Read the model definition and answer for the solid it produces. Units are mm, in the model's axes. A direction names the side the tool comes from. Coordinates: 2 decimals unless noted, no trailing zeros. Write each loop counter-clockwise with the first axis right and the second up, starting at its lowest first coordinate (ties: lowest second). Pieces come first, ordered by that corner, then holes. Notation, with made-up numbers: M 70,26 L 78,26 A13 cw 78,41 Z; hole C 13,76.5 d7. An arc over 180 degrees is marked long. Write item = value, one per line.
from build123d import *

# Parameters (mm, degrees)
BOSS_EXTRUDE1_DEPTH = 5
CUT_EXTRUDE1_DEPTH  = 42.207887594
CUT_EXTRUDE2_REACH  = 43.822
SKETCH5_R           = 1.5
SKETCH6_W           = 0.6
SKETCH6_H           = 2
CUT_EXTRUDE3_DEPTH  = 0.6
SKETCH8_W           = 56.6
SKETCH8_H           = 2.4
BOSS_EXTRUDE2_DEPTH = 2
SKETCH9_W           = 45
SKETCH9_H           = 5
BOSS_EXTRUDE3_DEPTH = 3
FILLET1_START       = -3
FILLET1_DEPTH       = 10
FILLET1_2_DEPTH     = 3
FILLET2_R           = 1


with BuildPart() as part:
    # Sketch1 → Boss-Extrude1 (new, symmetric)
    with BuildSketch(Plane.XY):
        with BuildLine():
            Line((-26.3, 1), (-26.3, 0))
            Line((-26.3, 0), (26.3, 0))
            Line((26.3, 0), (26.3, 1))
            ThreePointArc((26.3, 1), (28.057359313, 5.242640687), (32.3, 7))
            Line((32.3, 7), (40.3, 7))
            Line((40.3, 7), (40.3, 4))
            Line((40.3, 4), (32.3, 4))
            ThreePointArc((32.3, 4), (30.178679656, 3.121320344), (29.3, 1))
            Line((29.3, 1), (29.3, -2))
            ThreePointArc((29.3, -2), (29.007106781, -2.707106781), (28.3, -3))
            Line((28.3, -3), (-28.3, -3))
            ThreePointArc((-28.3, -3), (-29.007106781, -2.707106781), (-29.3, -2))
            Line((-29.3, -2), (-29.3, 1))
            ThreePointArc((-29.3, 1), (-30.178679656, 3.121320344), (-32.3, 4))
            Line((-32.3, 4), (-40.3, 4))
            Line((-40.3, 4), (-40.3, 7))
            Line((-40.3, 7), (-32.3, 7))
            ThreePointArc((-32.3, 7), (-28.057359313, 5.242640687), (-26.3, 1))
        make_face()
    extrude(amount=BOSS_EXTRUDE1_DEPTH, both=True)

    # Sketch3 → Cut-Extrude1 (cut, through all)
    with BuildSketch(Plane(origin=(0, 0, 0), x_dir=(1, 0, 0), z_dir=(0, 1, 0))):
        with BuildLine():
            Line((-23.6, 1.4), (23.6, 1.4))
            ThreePointArc((23.6, 1.4), (25, 0), (23.6, -1.4))
            Line((23.6, -1.4), (-23.6, -1.4))
            ThreePointArc((-23.6, -1.4), (-25, 0), (-23.6, 1.4))
        make_face()
    extrude(amount=-CUT_EXTRUDE1_DEPTH, mode=Mode.SUBTRACT)

    # Sketch5 → Cut-Extrude2 (cut, up to next)
    with BuildSketch(Plane(origin=(0, 7, 0), x_dir=(1, 0, 0), z_dir=(0, 1, 0)), mode=Mode.PRIVATE) as cut_extrude2_sk1:
        with Locations(Location((-36.3, 0, 0), (0, 0, 180))):
            Circle(SKETCH5_R)
    cut_extrude2_tool1 = extrude(cut_extrude2_sk1.sketch, amount=-CUT_EXTRUDE2_REACH, mode=Mode.PRIVATE) & part.part
    # Sketch5 → Cut-Extrude2 (cut, up to next)
    with BuildSketch(Plane(origin=(0, 7, 0), x_dir=(1, 0, 0), z_dir=(0, 1, 0)), mode=Mode.PRIVATE) as cut_extrude2_sk2:
        with Locations(Location((36.3, 0, 0), (0, 0, 180))):
            Circle(SKETCH5_R)
    cut_extrude2_tool2 = extrude(cut_extrude2_sk2.sketch, amount=-CUT_EXTRUDE2_REACH, mode=Mode.PRIVATE) & part.part
    add(cut_extrude2_tool1.solids().sort_by_distance((-36.3, 7, 0))[0], mode=Mode.SUBTRACT)
    add(cut_extrude2_tool2.solids().sort_by_distance((36.3, 7, 0))[0], mode=Mode.SUBTRACT)

    # Sketch6 → Cut-Extrude3 (cut)
    with BuildSketch(Plane(origin=(0, 0, 0), x_dir=(1, 0, 0), z_dir=(0, 1, 0))):
        with Locations((-5.9, 4)):
            Rectangle(SKETCH6_W, SKETCH6_H)
        with Locations((-3.4, 4)):
            Rectangle(SKETCH6_W, SKETCH6_H)
        with Locations((3.4, 4)):
            Rectangle(SKETCH6_W, SKETCH6_H)
        with Locations((-8.4, 4)):
            Rectangle(SKETCH6_W, SKETCH6_H)
        with Locations((-10.9, 4)):
            Rectangle(SKETCH6_W, SKETCH6_H)
        with Locations((-13.4, 4)):
            Rectangle(SKETCH6_W, SKETCH6_H)
        with Locations((5.9, 4)):
            Rectangle(SKETCH6_W, SKETCH6_H)
        with Locations((8.4, 4)):
            Rectangle(SKETCH6_W, SKETCH6_H)
        with Locations((10.9, 4)):
            Rectangle(SKETCH6_W, SKETCH6_H)
        with Locations((13.4, 4)):
            Rectangle(SKETCH6_W, SKETCH6_H)
    extrude(amount=-CUT_EXTRUDE3_DEPTH, mode=Mode.SUBTRACT)

    # Sketch8 → Boss-Extrude2 (add)
    with BuildSketch(Plane.XZ.offset(3)):
        with Locations((0, 3.8)):
            Rectangle(SKETCH8_W, SKETCH8_H)
    extrude(amount=BOSS_EXTRUDE2_DEPTH)

    # Sketch9 → Boss-Extrude3 (add)
    with BuildSketch(Plane.XZ.offset(3)):
        with Locations((0, -7.5)):
            Rectangle(SKETCH9_W, SKETCH9_H)
    extrude(amount=-BOSS_EXTRUDE3_DEPTH)

    # Fillet1: read off the stored shape, not the designer's step
    # Fillet1 outline → Fillet1 (cut)
    with BuildSketch(Plane(origin=(0, 0, 0), x_dir=(1, 0, 0), z_dir=(0, 1, 0)).offset(FILLET1_START)):
        with BuildLine():
            Line((-22.5, 10), (-22.5, 7.5))
            ThreePointArc((-22.5, 7.5), (-21.767766953, 9.267766953), (-20, 10))
            Line((-20, 10), (-22.5, 10))
        make_face()
        with BuildLine():
            Line((22.5, 10), (20, 10))
            ThreePointArc((20, 10), (21.767766953, 9.267766953), (22.5, 7.5))
            Line((22.5, 7.5), (22.5, 10))
        make_face()
    extrude(amount=FILLET1_DEPTH, mode=Mode.SUBTRACT)

    # Fillet1 2 outline → Fillet1 2 (add)
    with BuildSketch(Plane(origin=(0, 0, 0), x_dir=(1, 0, 0), z_dir=(0, 1, 0)).offset(FILLET1_START)):
        with BuildLine():
            Line((-22.5, 5), (-22.5, 7.5))
            ThreePointArc((-22.5, 7.5), (-23.232233047, 5.732233047), (-25, 5))
            Line((-25, 5), (-22.5, 5))
        make_face()
        with BuildLine():
            ThreePointArc((25, 5), (23.232233047, 5.732233047), (22.5, 7.5))
            Line((22.5, 7.5), (22.5, 5))
            Line((22.5, 5), (25, 5))
        make_face()
    extrude(amount=FILLET1_2_DEPTH)

    # Fillet2
    fillet2_edges = [part.edges().sort_by_distance(p)[0] for p in [
        (-28.3, -5, 3.8),
        (28.3, -5, 3.8),
    ]]
    fillet(fillet2_edges, radius=FILLET2_R)


solid = part.part
Item 1: Find section C-C (y = 1.75). Determine the outline of the cut face in (x, z).
Worked answers:
outline = M -29.4,-5 L -26.35,-5 L -26.35,5 L -29.4,5 Z; M 26.35,-5 L 29.4,-5 L 29.4,5 L 26.35,5 Z
Item 2: Which of the six approach directions +Z, -Z, +X, -X, +Y, -Y give full straight-line access (tool end or side, diameter ignored) to faces 4 (the face through (-34, 4, 0)), 5 (the face through (32.8, 4.3, -5)), 6 (the face through (-31, 4, -5))?
Worked answers:
face_4 = +Z, -Z, -X, -Y
face_5 = -Z, +X, +Y, -Y
face_6 = -Z, -X, +Y, -Y
Item 3: Find section B-B (z = 0). State how many separate pieces and enclosed holes the cut face has, and give its area (3 significant figures).
Worked answers:
separate_pieces = 4
enclosed_holes = 0
area = 104 mm²
Item 4: Find section A-A (x = 36.3). Determine the outline of the cut face in (y, z).
Worked answers:
outline = M 4,-5 L 7,-5 L 7,-1.5 L 4,-1.5 Z; M 4,1.5 L 7,1.5 L 7,5 L 4,5 Z
Item 5: Flat-ended cylindrical pins translate along their axes: pin 1 (6 mm diameter, centred on x = -14, z = 1.5, fed in from -Y); pin 2 (1.1 mm diameter, centred on y = 0.5, z = -2, fed in from -X); pin 3 (2.5 mm diameter, centred on x = 35.5, z = -1.5, fed in from -Y); pin 4 (6 mm diameter, centred on y = -1, z = -1, fed in from -X). Find the tip coordinate at first contact, or state that the pin passes through.
Worked answers:
pin_1 = -5
pin_2 = -29.3
pin_3 = 4
pin_4 = -29.47
Item 6: Consider line 1 along Z through (x, y) = (36.3, 4.85); line 2 along Y through (x, z) = (37, 2.25); line 3 along X through (y, z) = (0.75, 2). Determine where each line is inside the solid, lowest interval first. Write a range as from..to.
Worked answers:
line_1 = -5..-1.5, 1.5..5
line_2 = 4..7
line_3 = -29.3..-26.3, 26.3..29.3
Item 7: Find section D-D (x = -4.5). Determine the outline of the cut face in (y, z), and give its area (3 significant figures).
Worked answers:
outline = M -5,2.6 L -3,2.6 L -3,1.4 L 0,1.4 L 0,5 L -5,5 Z; M -3,-10 L 0,-10 L 0,-1.4 L -3,-1.4 Z
area = 41.4 mm²
Item 8: For a pull along Z with two mould halves and no side action, classify faces 1 (the face through (-40.3, 5, 0)), 2 (the face through (-37.73, 5.52, 0.45)), 3 (the face through (0, -4, 2.6)) as released by +Z, released by -Z, zero draft, split by the parting line, or undercut.
Worked answers:
face_1 = zero draft
face_2 = undercut
face_3 = released by -Z
